from build123d import *

# Parameters (mm, degrees)
SKETCH_1_W          = 41
SKETCH_1_H          = 10
EXTRUDE_1_DEPTH     = 2
SKETCH_2_W          = 41
SKETCH_2_H          = 5
EXTRUDE_2_DEPTH     = 2
SKETCH_3_R          = 1.25
CUT_EXTRUDE_1_DEPTH = 28.728178021


with BuildPart() as part:
    # 草圖1 → 填料-伸長1 (new body)
    with BuildSketch(Plane.XY):
        with Locations((4.676919413, 5.90754717)):
            Rectangle(SKETCH_1_W, SKETCH_1_H)
    extrude(amount=EXTRUDE_1_DEPTH)

    # 草圖2 → 填料-伸長2 (add)
    with BuildSketch(Plane.XY.offset(2)):
        with Locations((4.676919413, 3.40754717)):
            Rectangle(SKETCH_2_W, SKETCH_2_H)
    extrude(amount=EXTRUDE_2_DEPTH)

    # 草圖3 → 除料-伸長1 (cut, through all)
    with BuildSketch(Plane.XY.offset(4)):
        with Locations((-13.323080587, 3.40754717)):
            Circle(SKETCH_3_R)
        with Locations((22.676919413, 3.40754717)):
            Circle(SKETCH_3_R)
    extrude(amount=-CUT_EXTRUDE_1_DEPTH, mode=Mode.SUBTRACT)


solid = part.part
For this review, take the finished solid that the model builds, in its own axes (mm). A direction names the side the tool comes from. Round coordinates to 2 decimals unless told otherwise and drop trailing zeros. Loops run counter-clockwise (first coordinate to the right, second up) from the corner with the lowest first, then second, coordinate; pieces in that order, holes last. Notation, with made-up numbers: (-20, 47) - (14, 47) arc R21 ccw to (14, 86) - close; hole circle Ø11 at (56, 57.25). An arc over 180 degrees is marked (long way). Use one line per item in the form item = value.
1) We need section B-B on z = 2.75. Write out the cut boundary in (x, y).
Solutions:
outline = (-15.82, 0.91) - (25.18, 0.91) - (25.18, 5.91) - (-15.82, 5.91) - close; hole circle Ø2.5 at (-13.32, 3.41); hole circle Ø2.5 at (22.68, 3.41)
2) Mouldability with a two-part tool opening along X and no side actions: class faces 1 (the face through (4, 6, 0)), 2 (the face through (25.177, 5, 2)), 3 (the face through (21.43, 3.46, 2.03)) as pulls with the +X half, pulls with the -X half, needs draft (parallel to the pull), parting line crosses it, or undercut.
Solutions:
face_1 = needs draft
face_2 = pulls with the +X half
face_3 = undercut
3) We need section D-D on y = 9.5. Write out the cut boundary in (x, z), then the cut area to 3 significant figures.
Solutions:
outline = (-15.82, 0) - (25.18, 0) - (25.18, 2) - (-15.82, 2) - close
area = 82.0 mm2
4) We need section A-A on y = 3. Write out the cut boundary in (x, z).
Solutions:
outline = (-15.82, 0) - (-14.5, 0) - (-14.5, 4) - (-15.82, 4) - close; (-12.14, 0) - (21.5, 0) - (21.5, 4) - (-12.14, 4) - close; (23.86, 0) - (25.18, 0) - (25.18, 4) - (23.86, 4) - close
5) Clearance check with flat-ended pins moving along their axes: P1, Ø1.5, axis at x = 22.68, y = 3.41, coming from the -Z side; P2, Ø4, axis at x = 7, y = 6, coming from the +Z side; P3, Ø1, axis at x = 6.5, z = 3, coming from the +Y side; P4, Ø2.5, axis at x = 0.5, y = 7.5, coming from the +Z side. State where each tip first meets the part, or that it passes through.
Solutions:
P1 = through
P2 = 4
P3 = 5.91
P4 = 2
6) Wall thickness on probe 1 along X at (y, z) = (3.25, 0.85); probe 2 along X at (y, z) = (4.25, 3.35); probe 3 along Y at (x, z) = (-8, 3.6): over which ranges is each line inside the solid? List them lowest first.
Solutions:
probe_1 = -15.82 to -14.56, -12.08 to 21.44, 23.92 to 25.18
probe_2 = -15.82 to -14.25, -12.4 to 21.75, 23.6 to 25.18
probe_3 = 0.91 to 5.91
7) We need section C-C on x = -7.5. Write out the cut boundary in (y, z), then the cut area to 3 significant figures.
Solutions:
outline = (0.91, 0) - (10.91, 0) - (10.91, 2) - (5.91, 2) - (5.91, 4) - (0.91, 4) - close
area = 30.0 mm2
8) Tool access review of faces 4 (the face through (-15.823, 5, 2)), 5 (the face through (4, 5.908, 3)): name each direction out of +Z, -Z, +X, -X, +Y, -Y from which nothing blocks a thin tool from reaching the whole face with its end or side.
Solutions:
face_4 = +Z, -Z, -X, +Y, -Y
face_5 = +Z, +X, -X, +Y
